Geometry check sheet. Reference: the model listing, model coordinates, mm. Round coordinates to 2 decimals unless told otherwise and drop trailing zeros. Order: outer loops, then holes, each group sorted by start corner. A loop starts at its lowest first (then second) coordinate and runs counter-clockwise, first axis right, second up.
(1) Material ranges on line 1 along Y through (x, z) = (32.75, -4.75); line 2 along Y through (x, z) = (-6.25, 26.55); line 3 along Y through (x, z) = (31.35, -16.75), recorded low to high.
(2) Sectioned sample at B-B (y = 17). Record the boundary of the cut face in (x, z).
(3) Sectioned sample at C-C (z = 26). Give the number of separate pieces and of enclosed holes in the cut face, plus the area to 3 significant figures.
(4) Go/stop test with flat-tipped pins: pin 1 (3 mm diameter, centred on y = 0, z = 3.5, fed in from -X); pin 2 (3 mm diameter, centred on x = -17.5, y = 0, fed in from -Z). Record where each tip stops, or that it passes through.
(5) Sectioned sample at A-A (x = 3.5). Record the boundary of the cut face in (y, z).
(6) Release check for a two-part mould opening along Y. For faces 1 (the face through (30, 0, -5)), 2 (the face through (15, -20, 27)), 3 (the face through (-16.576, -0.383, 27.535)) record: +Y half, -Y half, draft (parallel to the pull), parting line (faces both ways), or undercut.
(7) Sectioned sample at D-D (z = 16). Record the boundary of the cut face in (x, y), plus the area to 3 significant figures.
from build123d import *

# Parameters (mm, degrees)
SKETCH1_W           = 70
SKETCH1_H           = 60
BOSS_EXTRUDE1_DEPTH = 20
SKETCH2_W           = 65
SKETCH2_H           = 55
CUT_EXTRUDE1_DEPTH  = 40
FILLET1_R           = 5
SKETCH3_R           = 1
CUT_EXTRUDE2_DEPTH  = 5
SKETCH4_R           = 1
CUT_EXTRUDE3_DEPTH  = 5


with BuildPart() as part:
    # Sketch1 → Boss-Extrude1 (new, symmetric)
    with BuildSketch(Plane(origin=(0, 0, 0), x_dir=(1, 0, 0), z_dir=(0, 1, 0))):
        Rectangle(SKETCH1_W, SKETCH1_H)
    extrude(amount=BOSS_EXTRUDE1_DEPTH, both=True)

    # Sketch2 → Cut-Extrude1 (cut)
    with BuildSketch(Plane(origin=(0, 20, 0), x_dir=(1, 0, 0), z_dir=(0, 1, 0))):
        with Locations((-2.5, 2.5)):
            Rectangle(SKETCH2_W, SKETCH2_H)
    extrude(amount=-CUT_EXTRUDE1_DEPTH, mode=Mode.SUBTRACT)

    # Fillet1
    fillet1_edges = [part.edges().sort_by_distance(p)[0] for p in [
        (30, 0, 25),
    ]]
    fillet(fillet1_edges, radius=FILLET1_R)

    # Sketch3 → Cut-Extrude2 (cut)
    with BuildSketch(Plane.XY.offset(30)):
        with Locations((-2.5, 0)):
            Circle(SKETCH3_R)
        with Locations((0.5, 0)):
            Circle(SKETCH3_R)
        with Locations((3.5, 0)):
            Circle(SKETCH3_R)
        with Locations((-6.25, -6.495190528)):
            Circle(SKETCH3_R)
        with Locations((-4.75, -9.09326674)):
            Circle(SKETCH3_R)
        with Locations((-3.25, -11.691342951)):
            Circle(SKETCH3_R)
        with Locations((-13.75, -6.495190528)):
            Circle(SKETCH3_R)
        with Locations((-15.25, -9.09326674)):
            Circle(SKETCH3_R)
        with Locations((-16.75, -11.691342951)):
            Circle(SKETCH3_R)
        with Locations((-17.5, 0)):
            Circle(SKETCH3_R)
        with Locations((-20.5, 0)):
            Circle(SKETCH3_R)
        with Locations((-23.5, 0)):
            Circle(SKETCH3_R)
        with Locations((-13.75, 6.495190528)):
            Circle(SKETCH3_R)
        with Locations((-15.25, 9.09326674)):
            Circle(SKETCH3_R)
        with Locations((-16.75, 11.691342951)):
            Circle(SKETCH3_R)
        with Locations((-6.25, 6.495190528)):
            Circle(SKETCH3_R)
        with Locations((-4.75, 9.09326674)):
            Circle(SKETCH3_R)
        with Locations((-3.25, 11.691342951)):
            Circle(SKETCH3_R)
    extrude(amount=-CUT_EXTRUDE2_DEPTH, mode=Mode.SUBTRACT)

    # Sketch4 → Cut-Extrude3 (cut)
    with BuildSketch(Plane(origin=(35, 0, 0), x_dir=(0, 0, -1), z_dir=(1, 0, 0))):
        with Locations((17.5, 0)):
            Circle(SKETCH4_R)
        with Locations((20.5, 0)):
            Circle(SKETCH4_R)
        with Locations((23.5, 0)):
            Circle(SKETCH4_R)
        with Locations((13.75, -6.495190528)):
            Circle(SKETCH4_R)
        with Locations((15.25, -9.09326674)):
            Circle(SKETCH4_R)
        with Locations((16.75, -11.691342951)):
            Circle(SKETCH4_R)
        with Locations((6.25, -6.495190528)):
            Circle(SKETCH4_R)
        with Locations((4.75, -9.09326674)):
            Circle(SKETCH4_R)
        with Locations((3.25, -11.691342951)):
            Circle(SKETCH4_R)
        with Locations((2.5, 0)):
            Circle(SKETCH4_R)
        with Locations((-0.5, 0)):
            Circle(SKETCH4_R)
        with Locations((-3.5, 0)):
            Circle(SKETCH4_R)
        with Locations((6.25, 6.495190528)):
            Circle(SKETCH4_R)
        with Locations((4.75, 9.09326674)):
            Circle(SKETCH4_R)
        with Locations((3.25, 11.691342951)):
            Circle(SKETCH4_R)
        with Locations((13.75, 6.495190528)):
            Circle(SKETCH4_R)
        with Locations((15.25, 9.09326674)):
            Circle(SKETCH4_R)
        with Locations((16.75, 11.691342951)):
            Circle(SKETCH4_R)
    extrude(amount=-CUT_EXTRUDE3_DEPTH, mode=Mode.SUBTRACT)


solid = part.part
Answer below:
1. line 1: y = -20 to -10.09, -8.09 to 8.09, 10.09 to 20
1. line 2: y = -20 to -7.5, -5.5 to 5.5, 7.5 to 20
1. line 3: y = -20 to -12.69, -10.69 to -0.66, 0.66 to 10.69, 12.69 to 20
2. outline: (-35, 25) - (25, 25) arc R5 cw to (30, 20) - (30, -30) - (35, -30) - (35, 30) - (-35, 30) - close
3. separate pieces: 1
3. enclosed holes: 18
3. area: 2,740 mm2
4. pin 1: stops at x = 30
4. pin 2: stops at z = 25
5. outline: (-20, 25) - (-1, 25) - (-1, 30) - (-20, 30) - close; (1, 25) - (20, 25) - (20, 30) - (1, 30) - close
6. face 1: draft
6. face 2: -Y half
6. face 3: undercut
7. outline: (30, -20) - (35, -20) - (35, 20) - (30, 20) - close
7. area: 200 mm2
